Autodesk Inventor part; units mm, degrees
ref_plane "YZ Plane" through (0, 0, 0) normal (1, 0, 0) x (0, 1, 0)
ref_plane "XZ Plane" through (0, 0, 0) normal (0, 1, 0) x (-1, 0, 0)
ref_plane "XY Plane" through (0, 0, 0) normal (0, 0, 1) x (1, 0, 0)
sketch "Sketch1" plane through (0, 0, 0) normal (0, 1, 0) x (-1, 0, 0)
  circle A0 centre (0, 0) radius 11
  dimension "d0" = 22
extrude "Extrusion1" add sketch "Sketch1" along normal blind 4
sketch "Sketch2" plane through (0, 4, 0) normal (0, 1, 0) x (1, 0, 0)
  circle A0 centre (-8, 0) radius 1
  point P0 (0, 0)
  dimension "d3" = 2
  dimension "d4" = 8
extrude "Extrusion2" cut sketch "Sketch2" against normal blind 10
pattern_circular "Circular Pattern1" count 4 over 360 about axis through (0, -10, 0) along (0, 1, 0) of "Extrusion2"
sketch "Sketch3" plane through (0, 4, 0) normal (0, 1, 0) x (1, 0, 0)
  line L0 (3.9, 3.9) -> (-3.9, 3.9)
  line L1 (-3.9, 3.9) -> (-3.9, -3.9)
  line L2 (-3.9, -3.9) -> (3.9, -3.9)
  line L3 (3.9, -3.9) -> (3.9, 3.9)
  line L4 (3.9, 3.9) -> (-3.9, -3.9) construction
  line L5 (-3.9, 3.9) -> (3.9, -3.9) construction
  line L6 (-3.9, -3.9) -> (-1.9, -3.9)
  line L7 (-1.9, -3.9) -> (-1.9, -1.9)
  line L8 (-1.9, -1.9) -> (-3.9, -1.9)
  line L9 (-3.9, -1.9) -> (-3.9, -3.9)
  line L10 (-3.9, 3.9) -> (-1.9, 3.9)
  line L11 (-1.9, 3.9) -> (-1.9, 1.9)
  line L12 (-1.9, 1.9) -> (-3.9, 1.9)
  line L13 (-3.9, 1.9) -> (-3.9, 3.9)
  line L14 (3.9, -3.9) -> (1.9, -3.9)
  line L15 (1.9, -3.9) -> (1.9, -1.9)
  line L16 (1.9, -1.9) -> (3.9, -1.9)
  line L17 (3.9, -1.9) -> (3.9, -3.9)
  line L18 (3.9, 3.9) -> (1.9, 3.9)
  line L19 (1.9, 3.9) -> (1.9, 1.9)
  line L20 (1.9, 1.9) -> (3.9, 1.9)
  line L21 (3.9, 1.9) -> (3.9, 3.9)
  point P0 (0, 0)
  point P1 (3.9, 1.9)
  point P2 (1.9, 3.9)
  point P3 (-1.9, 3.9)
  point P4 (-1.9, -3.9)
  point P5 (1.9, -3.9)
  dimension "d10" = 7.8
  dimension "d11" = 7.8
  dimension "d14" = 2
  dimension "d15" = 2
extrude "Extrusion3" add sketch "Sketch3" along normal blind 30 contours L19 L20 L3 L16 L15 L2 L7 L8 L1 L12 L11 L0
sketch "Sketch4" plane through (0, 34, 0) normal (0, 1, 0) x (1, 0, 0)
  circle A0 centre (0, 0) radius 0.75
  dimension "d16" = 1.5
extrude "Extrusion4" cut sketch "Sketch4" against normal blind 8
sketch "Sketch5" plane through (0, 0, 0) normal (0, -1, 0) x (1, 0, 0)
  circle A0 centre (0, 0) radius 0.75
  circle A1 centre (0, 0) radius 5
  dimension "d19" = 10
extrude "Extrusion5" cut sketch "Sketch5" against normal blind 2.2 contours A0 | A1
sketch "Sketch6" plane through (0, 2.2, 0) normal (0, -1, 0) x (1, 0, 0)
  circle A0 centre (0, 0) radius 2.5
  dimension "d22" = 5
extrude "Extrusion6" cut sketch "Sketch6" against normal blind 3
properties part number "XM430_motor_adaptor"
For this review, take the finished solid that the model builds, in its own axes (mm). A direction names the side the tool comes from. Round coordinates to 2 decimals unless told otherwise and drop trailing zeros. Write each loop counter-clockwise with the first axis right and the second up, starting at its lowest first coordinate (ties: lowest second). Pieces come first, ordered by that corner, then holes. Notation, with made-up numbers: M 4,11 L 63,11 A20 ccw 63,41 Z; hole C -20,87 d4. An arc over 180 degrees is marked long. One line per item, written item: value. Start each with the question number.
(1) We need section A-A (z = 0). Give the boundary of the cut face in (x, y).
(2) Insertion check: pin 1 (0.6 mm diameter, centred on y = 22, z = -3, fed in from +X); pin 2 (1.5 mm diameter, centred on x = -0.5, z = -0.5, fed in from -Y); pin 3 (1 mm diameter, centred on x = -2.5, y = 24, fed in from -Z); pin 4 (3 mm diameter, centred on x = 0, z = 8, fed in from -Y). Each pin has a flat end and moves straight along its axis. Give the tip position at first contact, or say it passes through.
(3) The part is to be moulded in two halves that separate along X. For faces 1 (the flat face through (-1, 34, 0)), 2 (the cylindrical face through (-1.08, 1.08, -4.88)), 3 (the flat face through (-3.9, 19, 0)), say which applies: released by +X, released by -X, zero draft, split by the parting line, or undercut.
(4) We need section C-C (y = 31). Give the boundary of the cut face in (x, z).
(5) Machinability: for faces 4 (the flat face through (-3, 19, 1.9)), 5 (the flat face through (0, 19, -3.9)), 6 (the flat face through (-1.9, 19, -3)), 7 (the cylindrical face through (-0.54, 3.68, -2.44)), 8 (the flat face through (3, 19, 1.9)), which of the approach directions +Z, -Z, +X, -X, +Y, -Y give a long, thin tool a straight path to every point of the face, cutting with its end or side? Answer none if there is none.
(6) We need section D-D (z = 7.75). Give the boundary of the cut face in (x, y), and give its area (3 significant figures).
(7) We need section B-B (x = 0). Give the boundary of the cut face in (y, z), and give its area (3 significant figures).
(8) Wall thickness on line 1 (X direction, y = 31, z = 0); line 2 (Z direction, x = -2.75, y = 29): over which ranges is each line inside the solid? List them lowest first.
Result:
1. outline: M -11,0 L -9,0 L -9,4 L -11,4 Z; M -7,0 L -5,0 L -5,2.2 L -2.5,2.2 L -2.5,5.2 L 2.5,5.2 L 2.5,2.2 L 5,2.2 L 5,0 L 7,0 L 7,4 L 3.9,4 L 3.9,34 L 0.75,34 L 0.75,26 L -0.75,26 L -0.75,34 L -3.9,34 L -3.9,4 L -7,4 Z; M 9,0 L 11,0 L 11,4 L 9,4 Z
2. pin 1: x = 1.9
2. pin 2: y = 5.2
2. pin 3: z = -1.9
2. pin 4: y = 0
3. face 1: zero draft
3. face 2: undercut
3. face 3: released by -X
4. outline: M -3.9,-1.9 L -1.9,-1.9 L -1.9,-3.9 L 1.9,-3.9 L 1.9,-1.9 L 3.9,-1.9 L 3.9,1.9 L 1.9,1.9 L 1.9,3.9 L -1.9,3.9 L -1.9,1.9 L -3.9,1.9 Z; hole C 0,0 d1.5
5. face 4: +Z, -X, +Y
5. face 5: -Z, +X, -X, +Y
5. face 6: -Z, -X, +Y
5. face 7: -Y
5. face 8: +Z, +X, +Y
6. outline: M -7.81,0 L -0.97,0 L -0.97,4 L -7.81,4 Z; M 0.97,0 L 7.81,0 L 7.81,4 L 0.97,4 Z
6. area: 54.7 mm²
7. outline: M 0,-11 L 4,-11 L 4,-9 L 0,-9 Z; M 0,-7 L 4,-7 L 4,-3.9 L 34,-3.9 L 34,-0.75 L 26,-0.75 L 26,0.75 L 34,0.75 L 34,3.9 L 4,3.9 L 4,7 L 0,7 L 0,5 L 2.2,5 L 2.2,2.5 L 5.2,2.5 L 5.2,-2.5 L 2.2,-2.5 L 2.2,-5 L 0,-5 Z; M 0,9 L 4,9 L 4,11 L 0,11 Z
7. area: 257 mm²
8. line 1: -3.9 to -0.75, 0.75 to 3.9
8. line 2: -1.9 to 1.9
